CAD build for the part. Positions are in the model's coordinates, mm. A direction names the side the tool comes from. Round coordinates to 2 decimals unless told otherwise and drop trailing zeros. Write each loop counter-clockwise with the first axis right and the second up, starting at its lowest first coordinate (ties: lowest second). Pieces come first, ordered by that corner, then holes. Notation, with made-up numbers: (24.25, 54) -> (28.25, 54) arc R21 ccw to (28.25, 68) -> close; hole circle Ø6 at (75, -3). An arc over 180 degrees is marked (long way). Answer in a Markdown table with one row per item. Add a question column.
```python
from build123d import *

# Parameters (mm, degrees)
BOSS_EXTRUDE1_DEPTH            = 8
CBORE_FOR_M5_SHCS1_D           = 5.5
CBORE_FOR_M5_SHCS1_DEPTH       = 8
CBORE_FOR_M5_SHCS1_CBORE_D     = 10.5
CBORE_FOR_M5_SHCS1_CBORE_DEPTH = 6
SKETCH6_R                      = 1
BOSS_EXTRUDE3_DEPTH            = 8
FILLET2_R                      = 1
BOSS_EXTRUDE4_DEPTH            = 3
BOSS_EXTRUDE4_DEPTH_BACK       = 8


with BuildPart() as part:
    # Sketch1 → Boss-Extrude1 (new body)
    with BuildSketch(Plane.XY):
        with BuildLine():
            Line((-17, -10), (17, -10))
            ThreePointArc((17, -10), (19.121320344, -9.121320344), (20, -7))
            Line((20, -7), (20, 10))
            Line((20, 10), (16, 10))
            ThreePointArc((16, 10), (15.292893219, 9.707106781), (15, 9))
            Line((15, 9), (15, 6))
            Line((15, 6), (5, 6))
            Line((5, 6), (5, 9))
            ThreePointArc((5, 9), (4.707106781, 9.707106781), (4, 10))
            Line((4, 10), (-20, 10))
            Line((-20, 10), (-20, -7))
            ThreePointArc((-20, -7), (-19.121320344, -9.121320344), (-17, -10))
        make_face()
    extrude(amount=BOSS_EXTRUDE1_DEPTH)

    # CBORE for M5 SHCS1
    with Locations(Plane.XY.offset(8)):
        with Locations((-10, 0), (10, 0)):
            CounterBoreHole(CBORE_FOR_M5_SHCS1_D / 2, CBORE_FOR_M5_SHCS1_CBORE_D / 2, CBORE_FOR_M5_SHCS1_CBORE_DEPTH, depth=CBORE_FOR_M5_SHCS1_DEPTH)

    # Sketch6 → Boss-Extrude3 (add)
    with BuildSketch(Plane.XY.offset(8)):
        with Locations((0, -2.727298247)):
            Circle(SKETCH6_R)
    extrude(amount=BOSS_EXTRUDE3_DEPTH)

    # Fillet2
    fillet2_edges = [part.edges().sort_by_distance(p)[0] for p in [
        (-1, -2.727298247, 16),
    ]]
    fillet(fillet2_edges, radius=FILLET2_R)

    # Sketch7 → Boss-Extrude4 (add, two sides)
    with BuildSketch(Plane.XY.offset(8)) as boss_extrude4_sk:
        with BuildLine():
            Line((20, -0.55), (15.221110993, -0.55))
            ThreePointArc((15.221110993, -0.55), (15.040589551, -1.467977174), (14.7, -2.339337513))
            Line((14.7, -2.339337513), (14.7, -10))
            Line((14.7, -10), (12.2, -10))
            Line((12.2, -10), (12.2, -10.5))
            Line((12.2, -10.5), (17, -10.5))
            ThreePointArc((17, -10.5), (19.121320344, -9.621320344), (20, -7.5))
            Line((20, -7.5), (20, -0.55))
        make_face()
    extrude(amount=BOSS_EXTRUDE4_DEPTH)
    extrude(boss_extrude4_sk.sketch, amount=-BOSS_EXTRUDE4_DEPTH_BACK)


solid = part.part
```
Item 1: Saw through at D-D on x = 0. Give the cut face in (y, z), then the cut area to 3 significant figures.
Item 2: Two-plate mould, pull along X, no slides. Class faces 1 (the cylindrical face through (-19.14, -9.1, 3.94)), 2 (the cylindrical face through (19.1, -9.64, 5.58)), 3 (the flat face through (18, 10, 4)), 4 (the cylindrical face through (15.301, 9.715, 3.944)): +X half, -X half, draft (parallel to the pull), parting line (faces both ways), or undercut.
Item 3: Pin check, flat tips, straight feed: pin 1 (6 mm diameter, centred on x = 15, y = -4, fed in from +Z); pin 2 (4 mm diameter, centred on x = 0.5, y = -1.5, fed in from +Z); pin 3 (0.9 mm diameter, centred on y = -6, z = 9, fed in from -X); pin 4 (4 mm diameter, centred on x = -7, z = 8, fed in from -Y). Stop position of each tip, or through.
Item 4: Saw through at B-B on z = 7. Give the cut face in (x, y).
Item 5: Saw through at C-C on x = -10. Give the cut face in (y, z), then the cut area to 3 significant figures.
Item 6: Saw through at A-A on y = 0. Give the cut face in (x, z).
Item 7: Drill centre lines: probe 1 along X at (y, z) = (8, 1.5); probe 2 along X at (y, z) = (-0.5, 7.25); probe 3 along Y at (x, z) = (10, 4.75). Where is each one in solid material? Low to high.
Item 8: Tool access for faces 5 (the flat face through (17, -5, 11)), 6 (the flat face through (5, 7, 4)), 7 (the flat face through (18, -0.55, 9)), 8 (the flat face through (-7.7, -2.3, 2)): list every direction of +Z, -Z, +X, -X, +Y, -Y with a clear straight run to the whole face (end or side of a thin tool).
Recorded:
| question | item | result |
|---|---|---|
| 1 | outline | (-10, 0) -> (10, 0) -> (10, 8) -> (-1.73, 8) -> (-1.73, 15) arc R1 ccw to (-3.73, 15) -> (-3.73, 8) -> (-10, 8) -> close |
| 1 | area | 176 mm2 |
| 2 | face 1 | -X half |
| 2 | face 2 | +X half |
| 2 | face 3 | draft |
| 2 | face 4 | undercut |
| 3 | pin 1 | z = 11 |
| 3 | pin 2 | z = 16 |
| 3 | pin 3 | x = 14.7 |
| 3 | pin 4 | y = -10 |
| 4 | outline | (-20, -7) arc R3 ccw to (-17, -10) -> (12.2, -10) -> (12.2, -10.5) -> (17, -10.5) arc R3 ccw to (20, -7.5) -> (20, 10) -> (16, 10) arc R1 ccw to (15, 9) -> (15, 6) -> (5, 6) -> (5, 9) arc R1 ccw to (4, 10) -> (-20, 10) -> close; hole circle Ø10.5 at (-10, 0); hole circle Ø10.5 at (10, 0) |
| 5 | outline | (-10, 0) -> (-2.75, 0) -> (-2.75, 2) -> (-5.25, 2) -> (-5.25, 8) -> (-10, 8) -> close; (2.75, 0) -> (10, 0) -> (10, 8) -> (5.25, 8) -> (5.25, 2) -> (2.75, 2) -> close |
| 5 | area | 86.0 mm2 |
| 6 | outline | (-20, 0) -> (-12.75, 0) -> (-12.75, 2) -> (-15.25, 2) -> (-15.25, 8) -> (-20, 8) -> close; (-7.25, 0) -> (7.25, 0) -> (7.25, 2) -> (4.75, 2) -> (4.75, 8) -> (-4.75, 8) -> (-4.75, 2) -> (-7.25, 2) -> close; (12.75, 0) -> (20, 0) -> (20, 8) -> (15.25, 8) -> (15.25, 2) -> (12.75, 2) -> close |
| 7 | probe 1 | -20 to 5, 15 to 20 |
| 7 | probe 2 | -20 to -15.23, -4.77 to 4.77, 15.23 to 20 |
| 7 | probe 3 | -10 to -5.25, 5.25 to 6 |
| 8 | face 5 | +Z, +X, +Y, -Y |
| 8 | face 6 | +Z, -Z, +Y |
| 8 | face 7 | +Z, +X, -X, +Y |
| 8 | face 8 | +Z |
